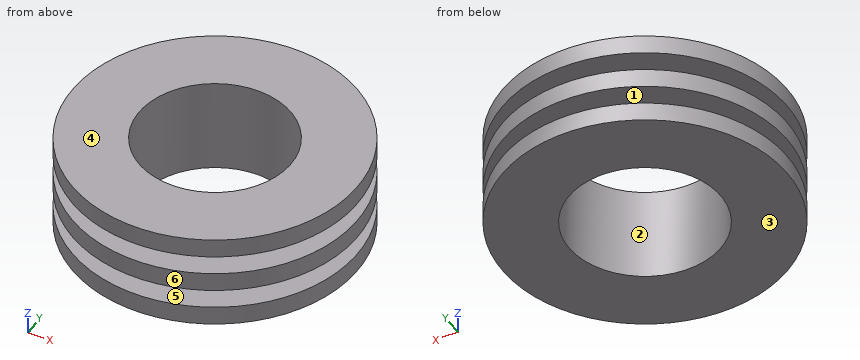
```python
from build123d import *

# Parameters (mm, degrees)
SKETCH_1_R      = 7.5
SKETCH_1_R_2    = 4
EXTRUDE_1_DEPTH = 5
SKETCH_2_W      = 1
SKETCH_2_H      = 1.5


with BuildPart() as part:
    # 草图1 → 凸台-拉伸1 (new body)
    with BuildSketch(Plane.XY):
        Circle(SKETCH_1_R)
        Circle(SKETCH_1_R_2, mode=Mode.SUBTRACT)
    extrude(amount=EXTRUDE_1_DEPTH)

    # 草图2 → 切除-旋转1 (revolve, cut)
    with BuildSketch(Plane(origin=(0, 0, 0), x_dir=(0, 0, -1), z_dir=(1, 0, 0)), mode=Mode.PRIVATE) as cut_revolve_1_sk:
        with Locations((-3.5, 6.75)):
            Rectangle(SKETCH_2_W, SKETCH_2_H)
        with Locations((-1.5, 6.75)):
            Rectangle(SKETCH_2_W, SKETCH_2_H)
    revolve(cut_revolve_1_sk.sketch.rotate(Axis((0, 0, 0), (0, 0, 1)), 90), axis=Axis((0, 0, 0), (0, 0, 1)), mode=Mode.SUBTRACT)


solid = part.part
```
Verification items for the finished model (mm, model axes). Face numbers are marked on the shaded views. A direction names the side the tool comes from. Coordinates: 2 decimals unless noted, no trailing zeros. Write each loop counter-clockwise with the first axis right and the second up, starting at its lowest first coordinate (ties: lowest second). Pieces come first, ordered by that corner, then holes. Notation, with made-up numbers: (65.5, 51.25) - (112.5, 51.25) arc R33 cw to (112.5, 80.25) - close; hole circle Ø3 at (-11, 89.25). An arc over 180 degrees is marked (long way). Write item = value, one per line.
Q1. Mould release check, pull along Z, two halves, no side actions. Record for the marked faces 1, 2, 3 and 4: released by +Z, released by -Z, zero draft, split by the parting line, or undercut.
Answer:
face_1 = undercut
face_2 = zero draft
face_3 = released by -Z
face_4 = released by +Z
Q2. Cross-section at C-C (z = 2.3). Enter the section's corners in (x, y).
Answer:
outline = circle Ø15 at (0, 0); hole circle Ø8 at (0, 0)
Q3. Access from +Z, -Z, +X, -X, +Y, -Y to the whole of each face (thin tool, end or side, straight path). Record for the marked faces 5 and 6.
Answer:
face_5 = none
face_6 = +Z, -Z
Q4. Go/stop test with flat-tipped pins: pin 1 Ø1.5 at (y, z) = (4, 3.5) entering from -X; pin 2 Ø1.5 at (x, y) = (-4.5, -2.5) entering from -Z. Record where each tip stops, or that it passes through.
Answer:
pin_1 = -6.66
pin_2 = 0
Q5. Cross-section at D-D (x = 5). Enter the section's corners in (y, z).
Answer:
outline = (-5.59, 0) - (5.59, 0) - (5.59, 1) - (3.32, 1) - (3.32, 2) - (5.59, 2) - (5.59, 3) - (3.32, 3) - (3.32, 4) - (5.59, 4) - (5.59, 5) - (-5.59, 5) - (-5.59, 4) - (-3.32, 4) - (-3.32, 3) - (-5.59, 3) - (-5.59, 2) - (-3.32, 2) - (-3.32, 1) - (-5.59, 1) - close
Q6. Material ranges on L1, parallel to Z at x = 5, y = 3.5; L2, parallel to Y at x = 0, z = 1.5; L3, parallel to Y at x = 0, z = 2.3, recorded low to high. Write a range as from..to.
Answer:
L1 = 0..1, 2..3, 4..5
L2 = -6..-4, 4..6
L3 = -7.5..-4, 4..7.5
Q7. Cross-section at A-A (x = 0). Enter the section's corners in (y, z).
Answer:
outline = (-7.5, 0) - (-4, 0) - (-4, 5) - (-7.5, 5) - (-7.5, 4) - (-6, 4) - (-6, 3) - (-7.5, 3) - (-7.5, 2) - (-6, 2) - (-6, 1) - (-7.5, 1) - close; (4, 0) - (7.5, 0) - (7.5, 1) - (6, 1) - (6, 2) - (7.5, 2) - (7.5, 3) - (6, 3) - (6, 4) - (7.5, 4) - (7.5, 5) - (4, 5) - close
